Here's how the part is built. I have some questions about the finished solid (model axes, mm). Face numbers are marked on the shaded views. Round coordinates to 2 decimals unless told otherwise and drop trailing zeros. Write each loop counter-clockwise with the first axis right and the second up, starting at its lowest first coordinate (ties: lowest second). Pieces come first, ordered by that corner, then holes. Notation, with made-up numbers: (56.25, -22) - (62.25, -22) arc R23 cw to (62.25, -3) - close; hole circle Ø4 at (75.5, 13). An arc over 180 degrees is marked (long way). One line per item, written item: value. Start each with the question number.
Item 1: Imagine slicing it at C-C, the plane y = 3. Please give me the cut outline in (x, z), then the cut area to 3 significant figures.
Item 2: If I drill on line 1 (X direction, y = 4.25, z = 0); line 2 (X direction, y = 5.5, z = -1.5), over which ranges is the centre line in solid material (lowest first)?
Item 3: Imagine slicing it at A-A, the plane z = 0. Please give me the cut outline in (x, y).
Item 4: Imagine slicing it at B-B, the plane x = 0. Please give me the cut outline in (y, z), then the cut area to 3 significant figures.
Item 5: Thinking about a two-plate mould opening in X: for the marked faces 1 and 2, which applies, released by +X, released by -X, zero draft, split by the parting line, or undercut?
Item 6: For P1, Ø6, axis at y = 5, z = -2.5, coming from the -X side; P2, Ø6, axis at y = 8.5, z = 4, coming from the -X side; P3, Ø2, axis at x = 7.5, y = 5, coming from the +Z side; P4, Ø0.9, axis at x = -10, y = 8, coming from the +Z side, each with a flat end and sliding along its axis, tell me the tip position at first contact or that it passes through.
```python
from build123d import *

# Parameters (mm, degrees)
SKETCH1_R           = 10.541
SKETCH1_R_2         = 9.398
BOSS_EXTRUDE1_DEPTH = 12.7
CUT_EXTRUDE1_DEPTH  = 12.7


with BuildPart() as part:
    # Sketch1 → Boss-Extrude1 (new body)
    with BuildSketch(Plane(origin=(0, 0, 0), x_dir=(1, 0, 0), z_dir=(0, 1, 0))):
        Circle(SKETCH1_R)
        Circle(SKETCH1_R_2, mode=Mode.SUBTRACT)
    extrude(amount=BOSS_EXTRUDE1_DEPTH)

    # Sketch2 → Cut-Extrude1 (cut)
    with BuildSketch(Plane(origin=(0, 0, 0), x_dir=(0, 0, -1), z_dir=(1, 0, 0))):
        with BuildLine():
            Line((-1.5875, 12.7), (1.5875, 12.7))
            Line((1.5875, 12.7), (1.5875, 6.35))
            ThreePointArc((1.5875, 6.35), (0, 4.7625), (-1.5875, 6.35))
            Line((-1.5875, 6.35), (-1.5875, 12.7))
        make_face()
    extrude(amount=-CUT_EXTRUDE1_DEPTH, mode=Mode.SUBTRACT)


solid = part.part
```
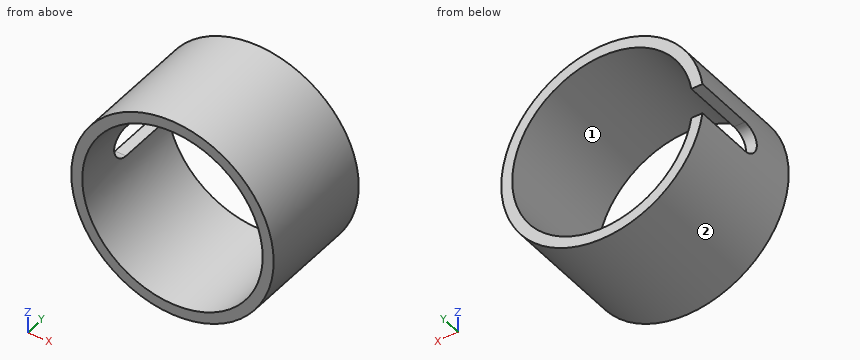
Values follow:
1. outline: circle Ø21.08 at (0, 0); hole circle Ø18.8 at (0, 0)
1. area: 71.6 mm^2
2. line 1: x = -10.54 to -9.4, 9.4 to 10.54
2. line 2: x = -10.43 to -9.28, 9.28 to 10.43
3. outline: (-10.54, 0) - (-9.4, 0) - (-9.4, 4.76) - (-10.54, 4.76) - close; (9.4, 0) - (10.54, 0) - (10.54, 12.7) - (9.4, 12.7) - close
4. outline: (0, -10.54) - (12.7, -10.54) - (12.7, -9.4) - (0, -9.4) - close; (0, 9.4) - (12.7, 9.4) - (12.7, 10.54) - (0, 10.54) - close
4. area: 29.0 mm^2
5. face 1: undercut
5. face 2: split by the parting line
6. P1: stops at x = -10.54
6. P2: stops at x = -10.42
6. P3: stops at z = 8.3
6. P4: stops at z = 4.46
